For this review, take the finished solid that the model builds, in its own axes (mm). Face numbers are marked on the shaded views. A direction names the side the tool comes from. Coordinates: 2 decimals unless noted, no trailing zeros. Loops run counter-clockwise (first coordinate to the right, second up) from the corner with the lowest first, then second, coordinate; pieces in that order, holes last. Notation, with made-up numbers: M -6.75,-14 L 7.25,-14 A14 ccw 7.25,13 Z; hole C 73.25,5.25 d7. An arc over 180 degrees is marked long. Put each result on its own line as item: value.
```python
from build123d import *

# Parameters (mm, degrees)
SKETCH1_R           = 3
BOSS_EXTRUDE1_DEPTH = 14
SKETCH2_R           = 1.2
BOSS_EXTRUDE2_DEPTH = 0.8
SKETCH3_R           = 0.4
BOSS_EXTRUDE3_DEPTH = 4.2
SKETCH4_R           = 0.3
BOSS_EXTRUDE4_DEPTH = 1


with BuildPart() as part:
    # Sketch1 → Boss-Extrude1 (new body)
    with BuildSketch(Plane(origin=(0, 0, 0), x_dir=(0, 0, -1), z_dir=(1, 0, 0))):
        Circle(SKETCH1_R)
    extrude(amount=BOSS_EXTRUDE1_DEPTH)

    # Sketch2 → Boss-Extrude2 (add)
    with BuildSketch(Plane.ZY):
        Circle(SKETCH2_R)
    extrude(amount=BOSS_EXTRUDE2_DEPTH)

    # Sketch3 → Boss-Extrude3 (add)
    with BuildSketch(Plane.ZY.offset(0.8)):
        Circle(SKETCH3_R)
    extrude(amount=BOSS_EXTRUDE3_DEPTH)

    # Sketch4 → Boss-Extrude4 (add)
    with BuildSketch(Plane(origin=(14, 0, 0), x_dir=(0, 0, -1), z_dir=(1, 0, 0))):
        with Locations((-2, 0)):
            Circle(SKETCH4_R)
        with Locations((2, 0)):
            Circle(SKETCH4_R)
    extrude(amount=BOSS_EXTRUDE4_DEPTH)


solid = part.part
```
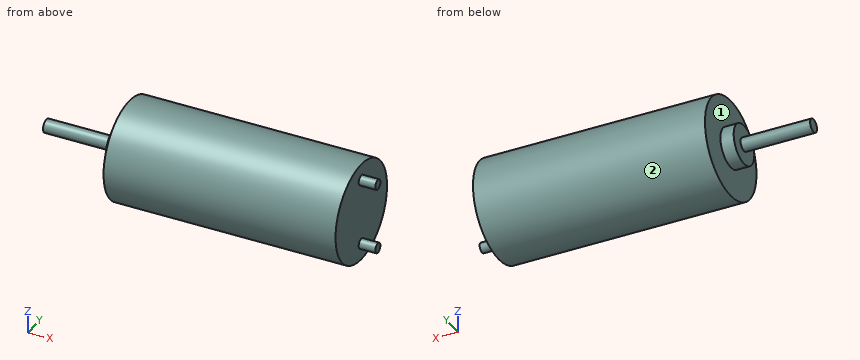
(1) Add section C-C (x = 4.25). Write out the cut boundary in (y, z), plus the area to 3 significant figures.
Determined:
outline: C 0,0 d6
area: 28.3 mm^2
(2) Add section D-D (z = -2). Write out the cut boundary in (x, y), plus the area to 3 significant figures.
Determined:
outline: M 0,-2.24 L 14,-2.24 L 14,-0.3 L 15,-0.3 L 15,0.3 L 14,0.3 L 14,2.24 L 0,2.24 Z
area: 63.2 mm^2
(3) Add section A-A (z = 0). Write out the cut boundary in (x, y).
Determined:
outline: M -5,-0.4 L -0.8,-0.4 L -0.8,-1.2 L 0,-1.2 L 0,-3 L 14,-3 L 14,3 L 0,3 L 0,1.2 L -0.8,1.2 L -0.8,0.4 L -5,0.4 Z
(4) For pin 1 (2 mm diameter, centred on y = 2, z = -2, fed in from +X); pin 2 (1 mm diameter, centred on x = 5.5, y = -2, fed in from -Z), all flat-tipped, find the tip position at first contact; note any pin that passes through.
Determined:
pin 1: stops at x = 14
pin 2: stops at z = -2.6
(5) Add section B-B (y = 0). Write out the cut boundary in (x, z).
Determined:
outline: M -5,-0.4 L -0.8,-0.4 L -0.8,-1.2 L 0,-1.2 L 0,-3 L 14,-3 L 14,-2.3 L 15,-2.3 L 15,-1.7 L 14,-1.7 L 14,1.7 L 15,1.7 L 15,2.3 L 14,2.3 L 14,3 L 0,3 L 0,1.2 L -0.8,1.2 L -0.8,0.4 L -5,0.4 Z
(6) Tool access review of the marked faces 1 and 2: name each direction out of +Z, -Z, +X, -X, +Y, -Y from which nothing blocks a thin tool from reaching the whole face with its end or side.
Determined:
face 1: -X
face 2: +X, -X
(7) Wall thickness on line 1 along X through (y, z) = (-0.4, 0.9); line 2 along Y through (x, z) = (8.5, 0.1); line 3 along X through (y, z) = (1.3, 2.2): over which ranges is each line inside the solid? List them lowest first. Write a range as [from, to].
Determined:
line 1: x = [-0.8, 14]
line 2: y = [-3, 3]
line 3: x = [0, 14]
